Verification items for the finished model (mm, model axes). Give positions to 0.01 mm unless a question says otherwise; leave off trailing zeros. Order: outer loops, then holes, each group sorted by start corner. A loop starts at its lowest first (then second) coordinate and runs counter-clockwise, first axis right, second up. Notation, with made-up numbers: (-19.75, 60) - (32.25, 60) arc R16 cw to (32.25, 65) - close; hole circle Ø7 at (41, -0.5). An arc over 180 degrees is marked (long way). Answer as a JSON object with one key per item and string values. Group by question number.
(1) Depth check by flat-ended pin: pin 1 Ø10 at (x, z) = (11, -2) entering from -Y; pin 2 Ø3 at (x, y) = (13, -24) entering from +Z; pin 3 Ø2 at (x, z) = (14, -33) entering from +Y (3 decimals). Enter the tip coordinate at first touch or a pass-through.
(2) Thickness scan on line 1 (Y direction, x = 4.5, z = 0); line 2 (Y direction, x = 12, z = 0); line 3 (Z direction, x = 1.75, y = -33). Record the ranges inside material, lowest first.
(3) Section check C-C (x = 10.75). Record the boundary of the cut face in (y, z), then the cut area to 3 significant figures.
(4) Section check A-A (y = 0). Record the boundary of the cut face in (x, z), then the cut area to 3 significant figures.
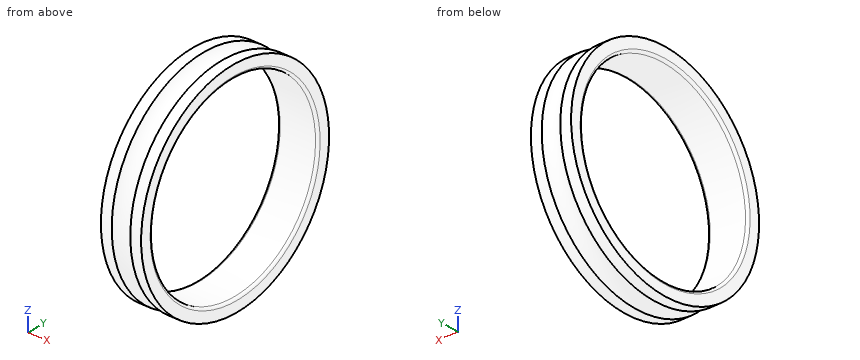
```python
from build123d import *


with BuildPart() as part:
    # Schizzo1 → Rivoluzione1 (revolve)
    with BuildSketch(Plane.XY, mode=Mode.PRIVATE) as rivoluzione1_sk:
        with BuildLine():
            Line((1.1, 42.5), (16.9, 42.5))
            ThreePointArc((16.9, 42.5), (17.677817459, 42.822182541), (18, 43.6))
            Line((18, 43.6), (18, 48.2))
            Line((18, 48.2), (13.161482939, 48.2))
            ThreePointArc((13.161482939, 48.2), (9, 46.0905), (4.838517061, 48.2))
            Line((4.838517061, 48.2), (0, 48.2))
            Line((0, 48.2), (0, 43.6))
            ThreePointArc((0, 43.6), (0.322182541, 42.822182541), (1.1, 42.5))
        make_face()
    revolve(rivoluzione1_sk.sketch.rotate(Axis((50, 0, 0), (-1, 0, 0)), 270), axis=Axis((50, 0, 0), (-1, 0, 0)))


solid = part.part
```
Solutions:
{
 "1": {"pin 1": "stops at y = -48.2", "pin 2": "stops at z = 42.62", "pin 3": "stops at y = 36.045"},
 "2": {"line 1": "y = -48.2 to -42.5, 42.5 to 48.2", "line 2": "y = -47.05 to -42.5, 42.5 to 47.05", "line 3": "z = -35.13 to -26.78, 26.78 to 35.13"},
 "3": {"outline": "circle Ø92.79 at (0, 0); hole circle Ø85 at (0, 0)", "area": "1,090 mm2"},
 "4": {"outline": "(0, -48.2) - (4.84, -48.2) arc R5.16 cw to (13.16, -48.2) - (18, -48.2) - (18, -43.6) arc R1.1 ccw to (16.9, -42.5) - (1.1, -42.5) arc R1.1 ccw to (0, -43.6) - close; (0, 43.6) arc R1.1 ccw to (1.1, 42.5) - (16.9, 42.5) arc R1.1 ccw to (18, 43.6) - (18, 48.2) - (13.16, 48.2) arc R5.16 cw to (4.84, 48.2) - (0, 48.2) - close", "area": "180 mm2"}
}
